Autodesk Fusion 360 part; units mm, degrees
sketch "Schizzo5" plane through (0, 0, 0) normal (0, 0, 1) x (1, 0, 0)
  line L0 (80.7173, 84.9147) -> (80.7173, -8.2853)
  circle A0 centre (85.7173, -5.7853) radius 1.5
  circle A1 centre (105.7173, 38.3147) radius 25 construction
  arc A2 (125.5163, 58.1137) -> (105.7173, 66.3147) centre (105.7173, 38.3147) ccw
  circle A3 centre (123.395, 55.9924) radius 3
  circle A4 centre (88.0397, 55.9924) radius 3
  arc A5 (105.7173, 66.3147) -> (85.9183, 58.1137) centre (105.7173, 38.3147) ccw
  circle A6 centre (125.7173, 82.4147) radius 3
  arc A7 (105.7173, 10.3147) -> (125.5163, 18.5157) centre (105.7173, 38.3147) ccw
  line L1 (80.7173, 38.3147) -> (130.7173, 38.3147) construction
  circle A8 centre (105.7173, 82.4147) radius 1.5
  circle A9 centre (85.7173, 82.4147) radius 3
  line L2 (105.7173, 38.3147) -> (123.395, 20.6371) construction
  arc A10 (105.7173, 66.3147) -> (85.9183, 58.1137) centre (105.7173, 38.3147) ccw
  circle A11 centre (85.7173, 82.4147) radius 1.5
  line L3 (130.7173, 84.9147) -> (80.7173, 84.9147)
  arc A12 (125.5163, 58.1137) -> (105.7173, 66.3147) centre (105.7173, 38.3147) ccw
  circle A13 centre (125.7173, 82.4147) radius 1.5
  line L4 (105.7173, 38.3147) -> (89.6274, 54.4047) construction
  circle A14 centre (105.7173, 82.4147) radius 3
  arc A15 (105.7173, 10.3147) -> (125.5163, 18.5157) centre (105.7173, 38.3147) ccw
  line L5 (105.7173, 38.3147) -> (105.7173, 13.3147) construction
  circle A16 centre (105.7173, 38.3147) radius 4.1
  circle A17 centre (105.7173, -5.7853) radius 1.5
  circle A18 centre (88.0397, 20.6371) radius 3
  line L6 (130.7173, -8.2853) -> (130.7173, 84.9147)
  arc A19 (85.9183, 18.5157) -> (105.7173, 10.3147) centre (105.7173, 38.3147) ccw
  line L7 (85.7173, 84.9147) -> (85.7173, -8.2853) construction
  arc A20 (105.7173, 13.3147) -> (123.395, 20.6371) centre (105.7173, 38.3147) ccw
  circle A21 centre (123.395, 20.6371) radius 3
  circle A22 centre (85.7173, -5.7853) radius 3
  circle A23 centre (105.7173, -5.7853) radius 3
  circle A24 centre (125.7173, -5.7853) radius 1.5
  line L8 (105.7173, 38.3147) -> (123.668, 56.2654) construction
  line L9 (80.7173, -8.2853) -> (130.7173, -8.2853)
  circle A25 centre (125.7173, -5.7853) radius 3
  line L10 (80.7173, -5.7853) -> (130.7173, -5.7853) construction
  line L11 (105.7173, 38.3147) -> (88.0397, 20.6371) construction
  arc A26 (85.9183, 18.5157) -> (105.7173, 10.3147) centre (105.7173, 38.3147) ccw
  line L12 (105.7173, 84.9147) -> (105.7173, -8.2853) construction
  arc A27 (88.0397, 20.6371) -> (105.7173, 13.3147) centre (105.7173, 38.3147) ccw
  line L13 (105.7173, 38.3147) -> (105.7173, 63.3147) construction
  line L14 (105.7173, 38.3147) -> (105.7173, 63.3147) construction
  line L15 (105.7173, 38.3147) -> (105.7173, 13.3147) construction
  arc A28 (105.7173, 16.3147) -> (121.2737, 22.7584) centre (105.7173, 38.3147) ccw
  arc A29 (90.161, 22.7584) -> (105.7173, 16.3147) centre (105.7173, 38.3147) ccw
  arc A30 (105.7173, 60.3147) -> (90.161, 53.8711) centre (105.7173, 38.3147) ccw
  arc A31 (121.2737, 53.8711) -> (105.7173, 60.3147) centre (105.7173, 38.3147) ccw
  dimension "d219" = 3
  dimension "d220" = 3
  dimension "d221" = 50
  dimension "d222" = 93.2
  dimension "d223" = 2.5
  dimension "d224" = 20
  dimension "d225" = 3
  dimension "d226" = 6
  dimension "d227" = 3
  dimension "d228" = 6
  dimension "d229" = 8.2
  dimension "d230" = 45
  dimension "d231" = 6
  dimension "d232" = 45
  dimension "d233" = 6
  dimension "d246" = -3
  dimension "d247" = -3
extrude "Estrusione24" add sketch "Schizzo5" along normal blind 5 contours L0 A6 A9 L3 A14 L6 A22 A23 L9 A25
extrude "Estrusione25" add sketch "Schizzo5" along normal blind 1.8 contours A9 L3 | A22 L9 | L3 A14 | A23 L9 | A6 L3 | L9 A25 picked at (85.7547, 84.58) picked at (85.7547, -7.9505) picked at (105.7547, 84.58) picked at (105.7547, -7.9505) picked at (125.7547, 84.58) picked at (125.7547, -7.9505)
equation "d225 = d227"
equation "d226 = d228"
Could you check a few things on this model? Use its own coordinates, in mm. A direction names the side the tool comes from. Coordinates: 2 decimals unless noted, no trailing zeros. Loops run counter-clockwise (first coordinate to the right, second up) from the corner with the lowest first, then second, coordinate; pieces in that order, holes last.
1. For P1, Ø3.5, axis at x = 105.72, y = -5.79, coming from the +Z side, with a flat end and sliding along its axis, tell me the tip position at first contact or that it passes through.
2. Imagine slicing it at A-A (y = 65). Please give me the cut outline in (x, z), and give its area (3 significant figures).
3. I need wall thicknesses on L1, parallel to Y at x = 106, z = 4.75; L2, parallel to Y at x = 94.5, z = 4.65; L3, parallel to Y at x = 88, z = 2.25. Which ranges of each line are inside material? Lowest first, please.
4. Imagine slicing it at C-C (z = 0.9). Give the number of separate pieces and of enclosed holes in the cut face, and give its area (3 significant figures).
5. We'd pull the mould along X, two halves only. Please class faces 1 (the face through (125.562, 53.918, 2.465)), 2 (the face through (80.717, 39, 2)), 3 (the face through (100, 39, 5)): released by +X, released by -X, zero draft, split by the parting line, or undercut.
6. Imagine slicing it at B-B (x = 95). Please give me the cut outline in (y, z).
7. Imagine slicing it at D-D (y = 37). Please give me the cut outline in (x, z).
8. For faces 4 (the face through (125.825, 79.417, 3.378)), 5 (the face through (130.717, 38, 2)), 6 (the face through (114.248, 18.036, 2.465)), which set-ups out of +Z, -Z, +X, -X, +Y, -Y let a thin tool reach every point of the face, with its end or its side?
Computed values:
1. P1: stops at z = 1.8
2. outline: (80.72, 0) - (97.24, 0) - (97.24, 5) - (80.72, 5) - close; (114.2, 0) - (130.72, 0) - (130.72, 5) - (114.2, 5) - close
2. area: 165 mm2
3. L1: y = -2.8 to 10.32, 16.32 to 34.22, 42.4 to 60.31, 66.31 to 79.43
3. L2: y = -8.29 to 12.66, 19.39 to 57.24, 63.97 to 84.91
3. L3: y = -8.29 to -7.73, -3.84 to 16.63, 23.64 to 52.99, 60 to 80.47, 84.36 to 84.91
4. separate pieces: 1
4. enclosed holes: 9
4. area: 4,040 mm2
5. face 1: undercut
5. face 2: released by -X
5. face 3: zero draft
6. outline: (-8.29, 0) - (12.45, 0) - (12.45, 5) - (-8.29, 5) - close; (19.1, 0) - (57.53, 0) - (57.53, 5) - (19.1, 5) - close; (64.18, 0) - (84.91, 0) - (84.91, 5) - (64.18, 5) - close
7. outline: (80.72, 0) - (101.83, 0) - (101.83, 5) - (80.72, 5) - close; (109.6, 0) - (130.72, 0) - (130.72, 5) - (109.6, 5) - close
8. face 4: +Z
8. face 5: +Z, -Z, +X, +Y, -Y
8. face 6: +Z, -Z
